Geometry: final body of the model. Coordinates: model frame, mm. A direction names the side the tool comes from. Give positions to 0.01 mm unless a question says otherwise; leave off trailing zeros. Write item = value, one per line. Start each with the question number.
from build123d import *

# Parameters (mm, degrees)
SKETCH_1_W      = 23.5
SKETCH_1_H      = 12
EXTRUDE_1_DEPTH = 771


with BuildPart() as part:
    # 草图1 → 凸台-拉伸1 (new, symmetric)
    with BuildSketch(Plane(origin=(0, 0, 0), x_dir=(0, 0, -1), z_dir=(1, 0, 0))):
        Polygon((-15, 15), (-11.5, 15), (-11.5, 13.5), (-11, 13.5), (-11, 12), (-9.5, 12), (-9.5, 15), (-8, 15), (-8, 12.5), (-5, 12.5), (-5, 15), (5, 15), (5, 12.5), (8, 12.5), (8, 15), (9.5, 15), (9.5, 12), (11, 12), (11, 13.5), (11.5, 13.5), (11.5, 15), (15, 15), (15, 8), (12.5, 8), (12.5, 5), (15, 5), (15, -5), (12.5, -5), (12.5, -8), (15, -8), (15, -15), (11.5, -15), (11.5, -13.5), (11, -13.5), (11, -12), (9.5, -12), (9.5, -15), (8, -15), (8, -12.5), (5, -12.5), (5, -15), (-5, -15), (-5, -12.5), (-8, -12.5), (-8, -15), (-9.5, -15), (-9.5, -12), (-11, -12), (-11, -13.5), (-11.5, -13.5), (-11.5, -15), (-15, -15), align=None)
        with BuildLine():
            Line((12, -10.5), (12, -8.5))
            ThreePointArc((12, -8.5), (11.853553391, -8.146446609), (11.5, -8))
            Line((11.5, -8), (-11.5, -8))
            ThreePointArc((-11.5, -8), (-11.853553391, -8.146446609), (-12, -8.5))
            Line((-12, -8.5), (-12, -10.5))
            ThreePointArc((-12, -10.5), (-11.853553391, -10.853553391), (-11.5, -11))
            Line((-11.5, -11), (11.5, -11))
            ThreePointArc((11.5, -11), (11.853553391, -10.853553391), (12, -10.5))
        make_face(mode=Mode.SUBTRACT)
        with BuildLine():
            Line((-11.5, 11), (11.5, 11))
            ThreePointArc((11.5, 11), (11.853553391, 10.853553391), (12, 10.5))
            Line((12, 10.5), (12, 8.5))
            ThreePointArc((12, 8.5), (11.853553391, 8.146446609), (11.5, 8))
            Line((11.5, 8), (-11.5, 8))
            ThreePointArc((-11.5, 8), (-11.853553391, 8.146446609), (-12, 8.5))
            Line((-12, 8.5), (-12, 10.5))
            ThreePointArc((-12, 10.5), (-11.853553391, 10.853553391), (-11.5, 11))
        make_face(mode=Mode.SUBTRACT)
        Rectangle(SKETCH_1_W, SKETCH_1_H, mode=Mode.SUBTRACT)
    extrude(amount=EXTRUDE_1_DEPTH, both=True)


solid = part.part
1) Access query for faces 3 (the flat face through (11, 0, 15)), 4 (the flat face through (11, -6, 0)). Directions: +Z, -Z, +X, -X, +Y, -Y. A direction counts if a zero-diameter tool reaches every point of the face in a straight line with its end or side. Return the directions, or none.
2) Cut plane A-A (x = 128). Give the number of separate pieces and of enclosed holes in the cut face, plus the area to 3 significant figures.
3) Pin query (flat end, axial travel): pin 1 Ø2.5 at (x, z) = (-337.5, 6.5) entering from -Y; pin 2 Ø0.6 at (x, z) = (43, -11) entering from +Y; pin 3 Ø1.6 at (x, z) = (-109.5, -10.5) entering from -Y; pin 4 Ø12 at (x, z) = (73.5, 6) entering from +Y. Return the tip coordinate at first contact, or that it passes through.
4) Ray query, L1, parallel to Y at x = -253, z = 2; L2, parallel to Y at x = -509, z = -10.75; L3, parallel to Z at x = 261, y = -13. Return the intervals inside material, ascending.
5) Draft query along Y for faces 1 (the flat face through (771, 7, 0)), 2 (the flat face through (11, 6, 0)). Return one class per face: pulls with the +Y half, pulls with the -Y half, needs draft (parallel to the pull), parting line crosses it, or undercut.
Reply:
q1.face_3 = +Z, +X, -X, +Y, -Y
q1.face_4 = +X, -X
q2.separate_pieces = 1
q2.enclosed_holes = 3
q2.area = 408 mm²
q3.pin_1 = -12.5
q3.pin_2 = 13.5
q3.pin_3 = -13.5
q3.pin_4 = 15
q4.L1 = -15 to -11, -8 to -6, 6 to 8, 11 to 15
q4.L2 = -12 to -11, -8 to -6, 6 to 8, 11 to 12
q4.L3 = -15 to -11, -9.5 to -8, -5 to 5, 8 to 9.5, 11 to 15
q5.face_1 = needs draft
q5.face_2 = undercut
